from build123d import *

# Parameters (mm, degrees)
F0_W     = 50.8
F0_H     = 31.75
F1_DEPTH = 101.6


# Not quite as in the source:
# - a feature names something its author has since deleted; it is built from what else it names
# - the program builds the solid bodies; features that only make, move or delete a surface that nothing else refers to are left out


with BuildPart() as f1:
    # F0 (on Front) → F1 (new body)
    with BuildSketch(Plane.XZ):
        with Locations((25.4, 15.875)):
            Rectangle(F0_W, F0_H)
    extrude(amount=-F1_DEPTH)

    # F5: sweep along a path in F2
    with BuildLine(Plane.XY.offset(31.75)) as f5_path:
        Line((50.8, 76.2), (50.8, 25.4))
        ThreePointArc((50.8, 25.4), (25.4, 0), (0, 25.4))
        Line((0, 25.4), (0, 76.2))
        ThreePointArc((0, 76.2), (25.4, 101.6), (50.8, 76.2))
    # F4 (on plane+point) → F5 (sweep, cut)
    with BuildSketch(Plane.XZ.offset(-25.4)):
        with BuildLine():
            Line((50.8, 21.59), (50.8, 31.75))
            Line((50.8, 31.75), (36.83, 31.75))
            add(Edge.make_bspline(
                [(50.8, 21.59), (50.8, 31.75), (36.83, 31.75)],
                knots=[0, 0, 0, 1.5707963268, 1.5707963268, 1.5707963268], degree=2, weights=[1, 0.7071067812, 1]))
        make_face()
        with BuildLine():
            Line((50.8, 0), (50.8, 10.16))
            add(Edge.make_bspline(
                [(36.83, 0), (50.8, 0), (50.8, 10.16)],
                knots=[4.7123889804, 4.7123889804, 4.7123889804, 6.2831853072, 6.2831853072, 6.2831853072], degree=2, weights=[1, 0.7071067812, 1]))
            Line((36.83, 0), (50.8, 0))
        make_face()
        Polygon((36.83, 31.75), (50.8, 31.75), (50.8, 21.59), (50.8, 10.16), (50.8, 0), (36.83, 0), (36.83, -19.05), (76.2, -19.05), (76.2, 10.16), (76.2, 21.59), (76.2, 50.8), (36.83, 50.8), align=None)
    sweep(path=f5_path.line, mode=Mode.SUBTRACT)


solid = f1.part
Verification items for the finished model (mm, model axes). Coordinates: 2 decimals unless noted, no trailing zeros. Order: outer loops, then holes, each group sorted by start corner. A loop starts at its lowest first (then second) coordinate and runs counter-clockwise, first axis right, second up.
1. Go/stop test with flat-tipped pins: pin 1 Ø1.5 at (y, z) = (76.5, 23.5) entering from -X; pin 2 Ø10 at (y, z) = (34, 8) entering from -X; pin 3 Ø4 at (y, z) = (85, 4) entering from +X; pin 4 Ø2 at (x, z) = (29.5, 4) entering from +Y. Record where each tip stops, or that it passes through.
Results found:
pin 1: stops at x = 0.09
pin 2: stops at x = 0
pin 3: stops at x = 48.1
pin 4: stops at y = 99.32
2. Sectioned sample at A-A, the plane z = 17. Record the cut outline in (x, y).
Results found:
outline: (0, 25.4) arc R25.4 ccw to (50.8, 25.4) - (50.8, 76.2) arc R25.4 ccw to (0, 76.2) - close
3. Scan lines: line 1 (X direction, y = 55, z = 10); line 2 (Z direction, x = 37, y = 39); line 3 (Y direction, x = 44, z = 12.5). Record each from-to range of solid material in increasing order.
Results found:
line 1: x = 0 to 50.8
line 2: z = 0 to 31.75
line 3: y = 8.1 to 93.5
